Autodesk Inventor part; units mm, degrees
ref_plane "YZ Plane" through (0, 0, 0) normal (1, 0, 0) x (0, 1, 0)
ref_plane "XZ Plane" through (0, 0, 0) normal (0, 1, 0) x (-1, 0, 0)
ref_plane "XY Plane" through (0, 0, 0) normal (0, 0, 1) x (1, 0, 0)
sketch "Sketch1" plane through (0, 0, 0) normal (1, 0, 0) x (0, 1, 0)
  line L0 (0, 12.5) -> (0, 0) construction
  line L1 (13, 0) -> (13, 28)
  line L2 (13, 28) -> (9.5, 28)
  line L3 (9.5, 28) -> (10.4778, 0)
  line L4 (13, 0) -> (10.4778, 0)
  dimension "d36" = 13
  dimension "d63" = 28
  dimension "d65" = 9.5
  dimension "d66" = 92
revolve "Revolution1" add sketch "Sketch1" angle 360 about axis through (0, 0, 12.5) along (0, 0, -1)
sketch "Sketch3" plane through (0, 0, 0) normal (1, 0, 0) x (0, 1, 0)
  line L0 (19, 0) -> (19, 28)
  line L1 (19, 28) -> (10.4778, 28)
  line L2 (19, 0) -> (10.4778, 0)
  line L3 (-10.4778, 0) -> (10.4778, 0)
  line L4 (10.4778, 0) -> (10.4778, 28)
  line L5 (-13, 28) -> (13, 28)
  point P0 (0, 0)
  dimension "d28" = 19
extrude "Extrusion1" add sketch "Sketch3" along normal mid plane 8
sketch "Sketch4" plane through (-4, 0, 0) normal (-1, 0, 0) x (0, 0, 1)
  circle A0 centre (10.5, 15.25) radius 1.6
  circle A1 centre (17.5, 15.25) radius 1.6
  line L0 (10.5, 15.25) -> (17.5, 15.25) construction
  line L1 (28, 19) -> (0, 19) construction
  circle A2 centre (24.5, 15.25) radius 1.6
  point P0 (0, 0)
  point P1 (17, 15.25)
  point P2 (14, 15.25)
  point P3 (14, 19)
  dimension "d29" = 3.2
  dimension "d30" = 3.2
  dimension "d31" = 7
  dimension "d34" = 3.75
  dimension "d67" = 3.2
  dimension "d68" = 7
extrude "Extrusion2" cut sketch "Sketch4" against normal blind 10
sketch "Sketch5" plane through (4, 0, 0) normal (1, 0, 0) x (0, 0, -1)
  circle A0 centre (-10.5, 15.25) radius 1.6
  circle A1 centre (-17.5, 15.25) radius 1.6
  line L0 (0, 12.3693) -> (-28, 12.3693)
  line L1 (-20.496, 19) -> (-21.5, 19)
  line L2 (-21.5, 19) -> (-21.5, 12.3693)
  line L3 (-21.5, 12.3693) -> (-20.496, 12.3693)
  line L4 (-20.496, 12.3693) -> (-20.496, 19)
  line L5 (0, 19) -> (-6.5, 19)
  line L6 (-6.5, 19) -> (-6.5, 12.3693)
  line L7 (-6.5, 12.3693) -> (0, 12.3693)
  line L8 (0, 12.3693) -> (0, 19)
  line L9 (0, 19) -> (-28, 19)
  point P0 (0, 0)
  dimension "d47" = 15
  dimension "d49" = 4
  dimension "d50" = 4
extrude "Extrusion3" cut sketch "Sketch5" against normal blind 10 contours L0 L6 L5 L8
equation "\"d49\" = d50"
properties part number "brush holder v5"
The model under review builds one solid part; all positions refer to its coordinate system, in mm. A direction names the side the tool comes from. Give positions to 0.01 mm unless a question says otherwise; leave off trailing zeros. Order: outer loops, then holes, each group sorted by start corner. A loop starts at its lowest first (then second) coordinate and runs counter-clockwise, first axis right, second up. Notation, with made-up numbers: (71, 8) - (101, 8) arc R28 ccw to (101, 31) - close; hole circle Ø5 at (8, -21). An arc over 180 degrees is marked (long way). Use CSV: the item, a comma, the result in double quotes. Start each with the question number.
Q1. Tool access review of faces 1 (the flat face through (-4, 17, 17)), 2 (the flat face through (4, 9, 28)), 3 (the cylindrical face through (-0.51, -12.99, 14.2)), 4 (the flat face through (0, 12.369, 3)), 5 (the flat face through (4, 17, 17)): name each direction out of +Z, -Z, +X, -X, +Y, -Y from which nothing blocks a thin tool from reaching the whole face with its end or side.
Q2. Clearance check with flat-ended pins moving along their axes: pin 1 Ø2 at (x, z) = (8.5, 7) entering from +Y; pin 2 Ø3 at (y, z) = (15.25, 10.5) entering from +X; pin 3 Ø7 at (x, z) = (-0.5, 1.5) entering from +Y; pin 4 Ø12 at (y, z) = (10.5, 7) entering from -X. State where each tip first meets the part, or that it passes through.
Q3. We need section A-A, the plane x = 0. Write out the cut boundary in (y, z), and give its area (3 significant figures).
Q4. The part is to be moulded in two halves that separate along Y. For faces 6 (the conical face through (-9.758, -2.167, 13.804)), 7 (the cylindrical face through (-0.056, 16.836, 24.292)), 8 (the flat face through (0, 16, 6.5)), 9 (the flat face through (0, 19, 17)), say which applies: +Y half, -Y half, draft (parallel to the pull), parting line (faces both ways), or undercut.
Q5. To check wall thickness, follow line 1 along X through (y, z) = (13, 11.25); line 2 along Y through (x, z) = (-0.25, 10.5); line 3 along Y through (x, z) = (0.75, 24.5). State the ranges of each line that lie inside material, in increasing order. Write a range as [from, to].
Q6. We need section B-B, the plane y = 0. Write out the cut boundary in (x, z).
Q7. We need section D-D, the plane y = 15.25. Write out the cut boundary in (x, z).
Q8. We need section C-C, the plane z = 17.5. Write out the cut boundary in (x, y), and give its area (3 significant figures).
Outcome:
1,face 1,"+Z, -Z, -X, +Y"
1,face 2,"+Z, +X, -X, +Y, -Y"
1,face 3,"+Z, -Z"
1,face 4,"-Z, +X, -X, +Y"
1,face 5,"+Z, -Z, +X, +Y"
2,pin 1,"stops at y = 10.62"
2,pin 2,"passes through"
2,pin 3,"stops at y = 12.37"
2,pin 4,"stops at x = -12.2"
3,outline,"(-13, 0) - (-10.48, 0) - (-9.5, 28) - (-13, 28) - close; (9.5, 28) - (10.48, 0) - (12.37, 0) - (12.37, 6.5) - (19, 6.5) - (19, 28) - close; hole circle Ø3.2 at (15.25, 10.5); hole circle Ø3.2 at (15.25, 17.5); hole circle Ø3.2 at (15.25, 24.5)"
3,area,"269 mm^2"
4,face 6,"undercut"
4,face 7,"undercut"
4,face 8,"draft"
4,face 9,"+Y half"
5,line 1,"x = [-4, 4]"
5,line 2,"y = [-13, -10.11], [10.11, 13.65], [16.85, 19]"
5,line 3,"y = [-12.98, -9.59], [9.59, 13.65], [16.85, 19]"
6,outline,"(-13, 0) - (-10.48, 0) - (-9.5, 28) - (-13, 28) - close; (9.5, 28) - (10.48, 0) - (13, 0) - (13, 28) - close"
7,outline,"(-4, 6.5) - (4, 6.5) - (4, 8.9) - (-4, 8.9) - close; (-4, 12.1) - (4, 12.1) - (4, 15.9) - (-4, 15.9) - close; (-4, 19.1) - (4, 19.1) - (4, 22.9) - (-4, 22.9) - close; (-4, 26.1) - (4, 26.1) - (4, 28) - (-4, 28) - close"
8,outline,"(-4, 12.37) arc R13 ccw (long way) to (4, 12.37) - (4, 13.65) - (-4, 13.65) - close; (-4, 16.85) - (4, 16.85) - (4, 19) - (-4, 19) - close; hole circle Ø19.73 at (0, 0)"
8,area,"249 mm^2"
